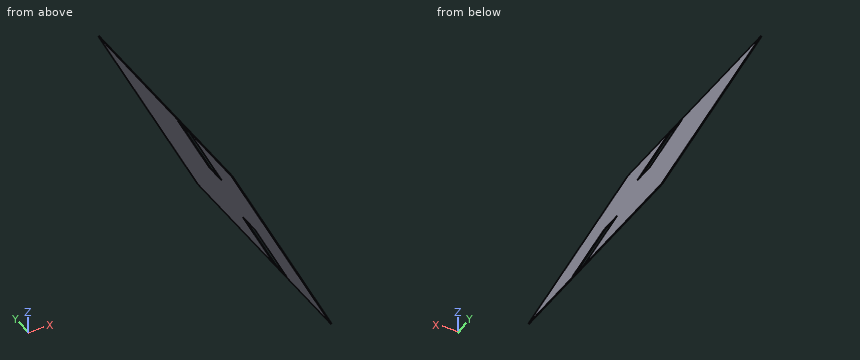
```python
from build123d import *

# Parameters (mm, degrees)
BOSS_EXTRUDE1_DEPTH = 6.35


with BuildPart() as part:
    # Sketch1 → Boss-Extrude1 (new body)
    with BuildSketch(Plane(origin=(-4014.627423578, 0, -2017.507429852), x_dir=(0.44902769125579206, 0, -0.8935178411679832), z_dir=(0.8935178411679832, 0, 0.44902769125579206))):
        Polygon((5982.803488378, 1987.55), (5036.653488378, 1987.55), (5036.653488378, 6.35), (5982.803488378, 6.35), (6928.953488378, 6.35), (6928.953488378, 1987.55), align=None)
        with BuildLine():
            Line((6293.953488378, 825.5), (6293.953488378, 647.7))
            ThreePointArc((6293.953488378, 647.7), (6295.813360317, 643.209871939), (6300.303488378, 641.35))
            Line((6300.303488378, 641.35), (6897.203488378, 641.35))
            ThreePointArc((6897.203488378, 641.35), (6901.693616438, 643.209871939), (6903.553488378, 647.7))
            Line((6903.553488378, 647.7), (6903.553488378, 825.5))
            ThreePointArc((6903.553488378, 825.5), (6901.693616438, 829.990128061), (6897.203488378, 831.85))
            Line((6897.203488378, 831.85), (6300.303488378, 831.85))
            ThreePointArc((6300.303488378, 831.85), (6295.813360317, 829.990128061), (6293.953488378, 825.5))
        make_face(mode=Mode.SUBTRACT)
        with BuildLine():
            Line((5068.403488378, 641.35), (5665.303488378, 641.35))
            ThreePointArc((5665.303488378, 641.35), (5669.793616438, 643.209871939), (5671.653488378, 647.7))
            Line((5671.653488378, 647.7), (5671.653488378, 825.5))
            ThreePointArc((5671.653488378, 825.5), (5669.793616438, 829.990128061), (5665.303488378, 831.85))
            Line((5665.303488378, 831.85), (5068.403488378, 831.85))
            ThreePointArc((5068.403488378, 831.85), (5063.913360317, 829.990128061), (5062.053488378, 825.5))
            Line((5062.053488378, 825.5), (5062.053488378, 647.7))
            ThreePointArc((5062.053488378, 647.7), (5063.913360317, 643.209871939), (5068.403488378, 641.35))
        make_face(mode=Mode.SUBTRACT)
    extrude(amount=-BOSS_EXTRUDE1_DEPTH)


solid = part.part
```
Build history of the part. All positions in model axes, mm. Coordinates: 2 decimals unless noted, no trailing zeros. Order: outer loops, then holes, each group sorted by start corner. A loop starts at its lowest first (then second) coordinate and runs counter-clockwise, first axis right, second up. Notation, with made-up numbers: (25, -22.5) -> (54, -22.5) arc R23 ccw to (54, 6.5) -> close; hole circle Ø11 at (-24.5, 17.25). An arc over 180 degrees is marked (long way). Answer in a Markdown table with one row per item. Add a question column.
Q1. Wall check: line 1 along Z through (x, y) = (-977, 1208); line 2 along Z through (x, y) = (-1679, 1902.5); line 3 along X through (y, z) = (905, -7389.5). Give the ranges that are in metal, low to high. Write a range as [from, to].
Q2. Drop flat-ended pins along their axis: pin 1 (12 mm diameter, centred on y = 499.5, z = -7909, fed in from +X); pin 2 (6 mm diameter, centred on y = 1493.5, z = -6692, fed in from -X); pin 3 (2 mm diameter, centred on x = -1617.5, y = 885, fed in from +Z); pin 4 (12 mm diameter, centred on x = -1600, z = -6802, fed in from +Y). Give the stop position or say it passes through.
Q3. Band-saw the part on A-A, the plane y = 782. List the corners of the cut face in (x, z), then the cut area to 3 significant figures.
Q4. Band-saw the part on B-B, the plane z = -6855. List the corners of the cut face in (x, y).
Q5. Band-saw the part on D-D, the plane y = 1562.5. List the corners of the cut face in (x, z).
Q6. Band-saw the part on C-C, the plane x = -1024.5. List the corners of the cut face in (y, z), then the cut area to 3 significant figures.
Answers follow:
| question | item | result |
|---|---|---|
| 1 | line 1 | [-8076.21, -8062.07] |
| 1 | line 2 | [-6679.3, -6665.16] |
| 1 | line 3 | [-1322.1, -1314.99] |
| 2 | pin 1 | x = -1050.91 |
| 2 | pin 2 | x = -1674.13 |
| 2 | pin 3 | z = -6785.55 |
| 2 | pin 4 | through |
| 3 | outline | (-1758.7, -6520.7) -> (-1747.3, -6543.39) -> (-1741.63, -6540.54) -> (-1753.03, -6517.85) -> close; (-1473.57, -7088.08) -> (-1194.14, -7644.12) -> (-1188.47, -7641.27) -> (-1467.9, -7085.23) -> close; (-920.41, -8188.81) -> (-909.01, -8211.5) -> (-903.34, -8208.65) -> (-914.74, -8185.96) -> close |
| 3 | area | 4,270 mm^2 |
| 4 | outline | (-1590.7, 6.35) -> (-1583.6, 6.35) -> (-1583.6, 641.35) -> (-1590.7, 641.35) -> close; (-1590.7, 831.85) -> (-1583.6, 831.85) -> (-1583.6, 1987.55) -> (-1590.7, 1987.55) -> close |
| 5 | outline | (-1758.7, -6520.7) -> (-909.01, -8211.5) -> (-903.34, -8208.65) -> (-1753.03, -6517.85) -> close |
| 6 | outline | (6.35, -7981.69) -> (641.35, -7981.69) -> (641.35, -7967.55) -> (6.35, -7967.55) -> close; (831.85, -7981.69) -> (1987.55, -7981.69) -> (1987.55, -7967.55) -> (831.85, -7967.55) -> close |
| 6 | area | 25,300 mm^2 |
